Input: part model. Units: mm. Frame: model coordinates. Coordinates: 2 decimals unless noted, no trailing zeros. Write each loop counter-clockwise with the first axis right and the second up, starting at its lowest first coordinate (ties: lowest second). Pieces come first, ordered by that corner, then holes. Notation, with made-up numbers: (60.5, 65.25) - (113.5, 65.25) arc R18 cw to (113.5, 78.25) - close; hole circle Ø10 at (58, 83). An arc over 180 degrees is marked (long way). Use CSV: the item, a comma, the result in double quotes.
```python
from build123d import *

# Parameters (mm, degrees)
BOSS_EXTRUDE1_DEPTH    = 381
F_10_CLEARANCE_HOLE1_D = 5.1054


with BuildPart() as part:
    # Sketch1 → Boss-Extrude1 (new body)
    with BuildSketch(Plane(origin=(0, 0, 0), x_dir=(1, 0, 0), z_dir=(0, 1, 0))):
        Polygon((7.332348419, 0), (3.666174209, 6.35), (-3.666174209, 6.35), (-7.332348419, 0), (-3.666174209, -6.35), (3.666174209, -6.35), align=None)
    extrude(amount=BOSS_EXTRUDE1_DEPTH)

    # Sketch2 → Tap Drill for #10-24 Tap1 (revolve, cut)
    with BuildSketch(Plane(origin=(0, 381, 0), x_dir=(0, 0, 1), z_dir=(1, 0, 0))):
        Polygon((0, 0), (0, 26.540824014), (1.89865, 25.4), (1.89865, 0), align=None)
    tap_drill_for_10_24_tap1 = revolve(axis=Axis((0, 387.35, 0), (0, -1, 0)), mode=Mode.SUBTRACT)

    # Mirror1: Tap Drill for #10-24 Tap1 across plane
    add(tap_drill_for_10_24_tap1.mirror(Plane.ZX.offset(190.5)), mode=Mode.SUBTRACT)

    # #10 Clearance Hole1 (through all)
    with Locations(Plane(origin=(0, 0, -6.35), x_dir=(-1, 0, 0), z_dir=(0, 0, -1))):
        with Locations((0, 139.7), (0, 241.3)):
            Hole(F_10_CLEARANCE_HOLE1_D / 2)


solid = part.part
```
(1) Cut plane A-A on y = 39. Return loops of the section in (x, z), and give its area (3 significant figures).
Check values:
outline,"(-7.33, 0) - (-3.67, -6.35) - (3.67, -6.35) - (7.33, 0) - (3.67, 6.35) - (-3.67, 6.35) - close"
area,"140 mm^2"
(2) Pin query (flat end, axial travel): pin 1 Ø2.5 at (x, z) = (0, 0) entering from +Y; pin 2 Ø2.5 at (x, z) = (0, 0) entering from -Y; pin 3 Ø3 at (x, y) = (6, 279.5) entering from +Z. Return the tip coordinate at first contact, or that it passes through.
Check values:
pin 1,"y = 355.21"
pin 2,"y = 25.79"
pin 3,"z = 4.91"
(3) Ray query, probe 1 along Y at (x, z) = (-0.25, 4.25); probe 2 along Z at (x, y) = (0, 15.75); probe 3 along Y at (x, z) = (-0.25, -1). Return the intervals inside material, ascending. Write a range as from..to.
Check values:
probe 1,"0..137.16, 142.24..238.76, 243.84..381"
probe 2,"-6.35..-1.9, 1.9..6.35"
probe 3,"25.92..137.16, 142.24..238.76, 243.84..355.08"
